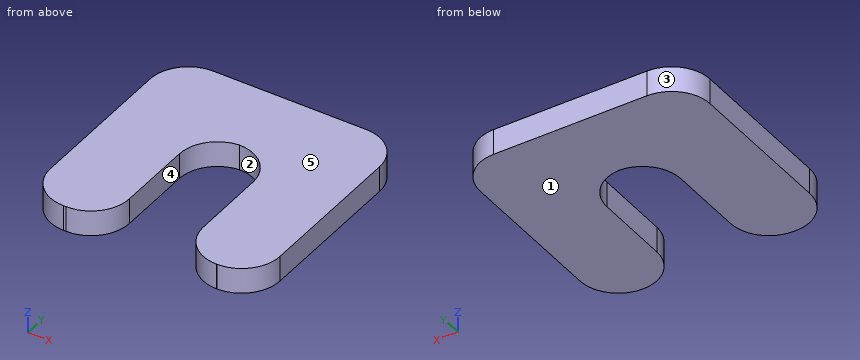
```python
from build123d import *

# Parameters (mm, degrees)
F1_DEPTH    = 10
F2_R        = 15
F3_R        = 15
F4_R        = 15
F5_R        = 15
F6_T1_DEPTH = 10


# Not quite as in the source:
# - a fillet or chamfer that OpenCascade refuses, or shapes differently, is made with other operations: its cross-section is extruded or revolved along the edge and cut away or added


with BuildPart() as f1:
    # F0 (on Top) → F1 (new body)
    with BuildSketch(Plane.XY):
        Polygon((0, 90), (0, 0), (30.9630036354, 0), (30.9630036354, 60), (59.8146165162, 60), (60, 0), (90, 0), (90, 90), align=None)
    extrude(amount=F1_DEPTH)

    # F2
    f2_edges = [f1.edges().sort_by_distance(p)[0] for p in [
        (0, 90, 5),
        (90, 90, 5),
    ]]
    fillet(f2_edges, radius=F2_R)

    # F3
    f3_edges = [f1.edges().sort_by_distance(p)[0] for p in [
        (0, 0, 5),
        (30.963004, 0, 5),
    ]]
    fillet(f3_edges, radius=F3_R)

    # F4
    f4_edges = [f1.edges().sort_by_distance(p)[0] for p in [
        (60, 0, 5),
        (90, 0, 5),
    ]]
    fillet(f4_edges, radius=F4_R)

    # F5
    f5_edges = [f1.edges().sort_by_distance(p)[0] for p in [
        (59.814617, 60, 5),
    ]]
    fillet(f5_edges, radius=F5_R)

    # F6: fillet of radius 15 on 1 edges, made by hand

    # F6_s2 → F6_t1 (join)
    with BuildSketch(Plane.XY):
        with BuildLine():
            ThreePointArc((44.8608907894, 60), (34.9736521375, 55.2500561159), (30.9630036354, 45.0405432159))
            Line((30.9630036354, 45.0405432159), (30.9630036354, 60))
            Line((30.9630036354, 60), (44.8608907894, 60))
        make_face()
    extrude(amount=F6_T1_DEPTH)


solid = f1.part
```
Geometry: final body of the model. Coordinates: model frame, mm. Face numbers are marked on the shaded views. A direction names the side the tool comes from. Give positions to 0.01 mm unless a question says otherwise; leave off trailing zeros. Write each loop counter-clockwise with the first axis right and the second up, starting at its lowest first coordinate (ties: lowest second). Pieces come first, ordered by that corner, then holes.
1. Section query A-A, the plane z = 5. Return loops of the section in (x, y), then the cut area to 3 significant figures.
2. Section query C-C, the plane y = 7.5. Return loops of the section in (x, z), then the cut area to 3 significant figures.
3. Section query D-D, the plane x = 35. Return loops of the section in (y, z), then the cut area to 3 significant figures.
4. Reachability of the marked faces 4 and 5 from +Z, -Z, +X, -X, +Y, -Y: full face, straight path, thin tool, end or side. Return the list, or none.
5. Pin query (flat end, axial travel): P1, Ø10, axis at x = 48.5, y = 68, coming from the -Z side. Return the tip coordinate at first contact, or that it passes through.
6. Line query: probe 1 along X at (y, z) = (38, 2.75); probe 2 along X at (y, z) = (11, 4.25); probe 3 along Y at (x, z) = (38, 5.5). Output: solid intervals per line, ascending.
7. Draft query along X for the marked faces 1, 2 and 3. Return one class per face: released by +X, released by -X, zero draft, split by the parting line, or undercut.
8. Section query B-B, the plane y = 37.5. Return loops of the section in (x, z).
Computed:
1. outline: (0, 15) arc R15 ccw to (15, 0) - (15.96, 0) arc R15 ccw to (30.96, 15) - (30.96, 45.04) arc R15 cw to (44.86, 60) arc R15 cw to (59.86, 45.05) - (59.95, 14.95) arc R15 ccw to (74.95, 0) - (75, 0) arc R15 ccw to (90, 15) - (90, 75) arc R15 ccw to (75, 90) - (15, 90) arc R15 ccw to (0, 75) - close
1. area: 6,170 mm2
2. outline: (2.01, 0) - (28.95, 0) - (28.95, 10) - (2.01, 10) - close; (61.96, 0) - (87.99, 0) - (87.99, 10) - (61.96, 10) - close
2. area: 530 mm2
3. outline: (55.28, 0) - (90, 0) - (90, 10) - (55.28, 10) - close
3. area: 347 mm2
4. face 4: +Z, -Z, -Y
4. face 5: +Z, +X, -X, +Y, -Y
5. P1: stops at z = 0
6. probe 1: x = 0 to 30.96, 59.88 to 90
6. probe 2: x = 0.54 to 30.42, 60.5 to 89.46
6. probe 3: y = 57.75 to 90
7. face 1: zero draft
7. face 2: undercut
7. face 3: released by -X
8. outline: (0, 0) - (30.96, 0) - (30.96, 10) - (0, 10) - close; (59.88, 0) - (90, 0) - (90, 10) - (59.88, 10) - close
